The figure shows three views and two pictorial views of one solid part (mm, origin at its lowest corner). Answer the questions. A direction names the side the tool comes from. Coordinates: 2 decimals unless noted, no trailing zeros. Write each loop counter-clockwise with the first axis right and the second up, starting at its lowest first coordinate (ties: lowest second). Pieces come first, ordered by that corner, then holes.
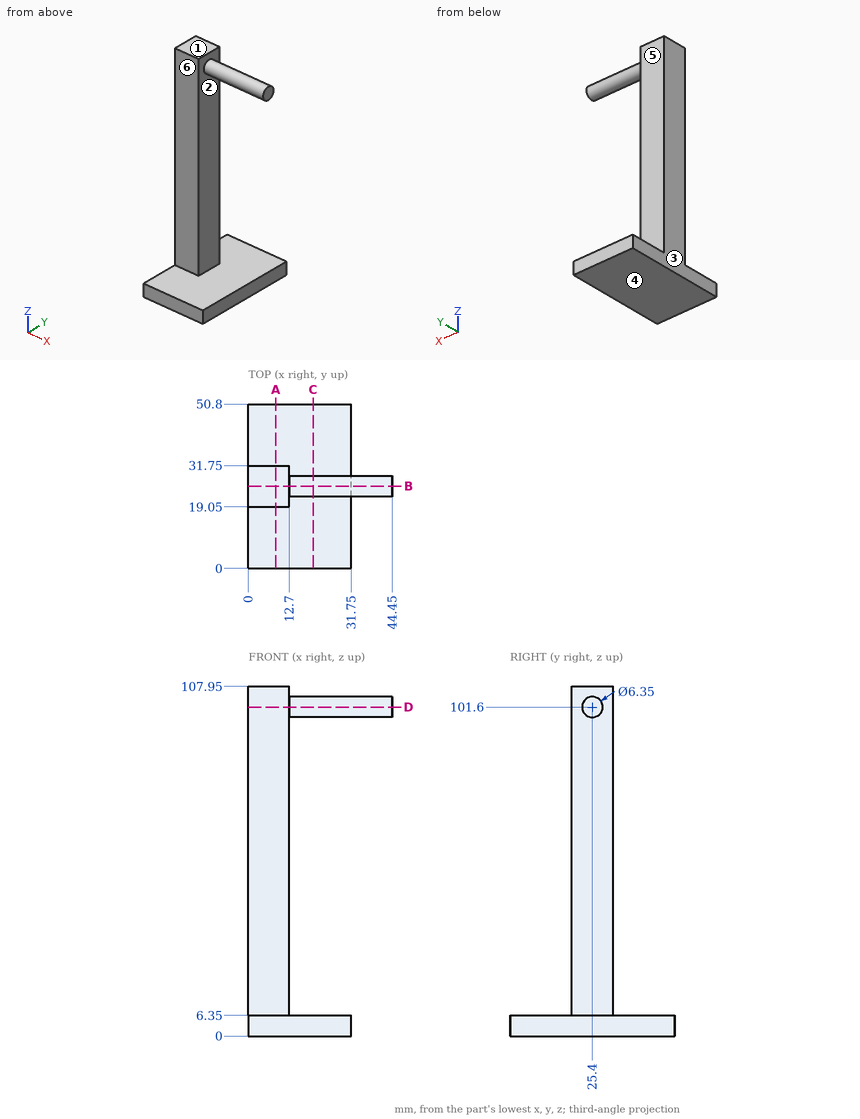
Item 1: For the marked faces 5 and 6, determine the directions among +Z, -Z, +X, -X, +Y, -Y from which every point of the face is accessible in a straight line to the end or side of a thin tool.
Item 2: The part is cut by section C-C (x = 20). Give the vertices of the cut face in (y, z) (3 decimals), and give its area (3 significant figures).
Item 3: Given pin 1 (5 mm diameter, centred on x = 29.5, y = 7.5, fed in from +Z); pin 2 (2 mm diameter, centred on x = 13, y = 26, fed in from -Z); pin 3 (10 mm diameter, centred on y = 25.5, z = 34.5, fed in from +X); pin 4 (4 mm diameter, centred on x = 9.5, z = 68.5, fed in from -Y), each flat-ended and moving along its own axis, determine where each tip first touches the part or whether it passes through.
Item 4: The part is cut by section A-A (x = 8.5). Give the vertices of the cut face in (y, z).
Item 5: The part is cut by section D-D (z = 101.6). Give the vertices of the cut face in (x, y) (3 decimals).
Item 6: The part is cut by section B-B (y = 25.4). Give the vertices of the cut face in (x, z) (3 decimals).
Item 7: Determine the mould class of the marked faces 1, 2, 3 and 4 for opening direction Z: +Z half, -Z half, draft (parallel to the pull), parting line (faces both ways), or undercut.
Item 8: Find the intervals of material crossed by probe 1 along X at (y, z) = (19.5, 103); probe 2 along Y at (x, z) = (5, 99.5); probe 3 along Z at (x, y) = (31, 20.5), in increasing order.
Answer:
1. face 5: +Z, +X, -X, +Y
1. face 6: +Z, +X, -X, -Y
2. outline: (0, 0) - (50.8, 0) - (50.8, 6.35) - (0, 6.35) - close; circle Ø6.35 at (25.4, 101.6)
2. area: 354 mm2
3. pin 1: stops at z = 6.35
3. pin 2: stops at z = 0
3. pin 3: stops at x = 12.7
3. pin 4: stops at y = 19.05
4. outline: (0, 0) - (50.8, 0) - (50.8, 6.35) - (31.75, 6.35) - (31.75, 107.95) - (19.05, 107.95) - (19.05, 6.35) - (0, 6.35) - close
5. outline: (0, 19.05) - (12.7, 19.05) - (12.7, 22.225) - (44.45, 22.225) - (44.45, 28.575) - (12.7, 28.575) - (12.7, 31.75) - (0, 31.75) - close
6. outline: (0, 0) - (31.75, 0) - (31.75, 6.35) - (12.7, 6.35) - (12.7, 98.425) - (44.45, 98.425) - (44.45, 104.775) - (12.7, 104.775) - (12.7, 107.95) - (0, 107.95) - close
7. face 1: +Z half
7. face 2: undercut
7. face 3: draft
7. face 4: -Z half
8. probe 1: x = 0 to 12.7
8. probe 2: y = 19.05 to 31.75
8. probe 3: z = 0 to 6.35
